Source: three-view drawing plus pictorial views. Frame: mm from the lowest corner of the part. Coordinates: 2 decimals unless noted, no trailing zeros. Loops run counter-clockwise (first coordinate to the right, second up) from the corner with the lowest first, then second, coordinate; pieces in that order, holes last. Notation, with made-up numbers: (59.5, 7) - (67.5, 7) arc R12 ccw to (67.5, 30) - close; hole circle Ø8 at (33.5, 15). An arc over 180 degrees is marked (long way). Return JSON: item names as keys, results as strings.
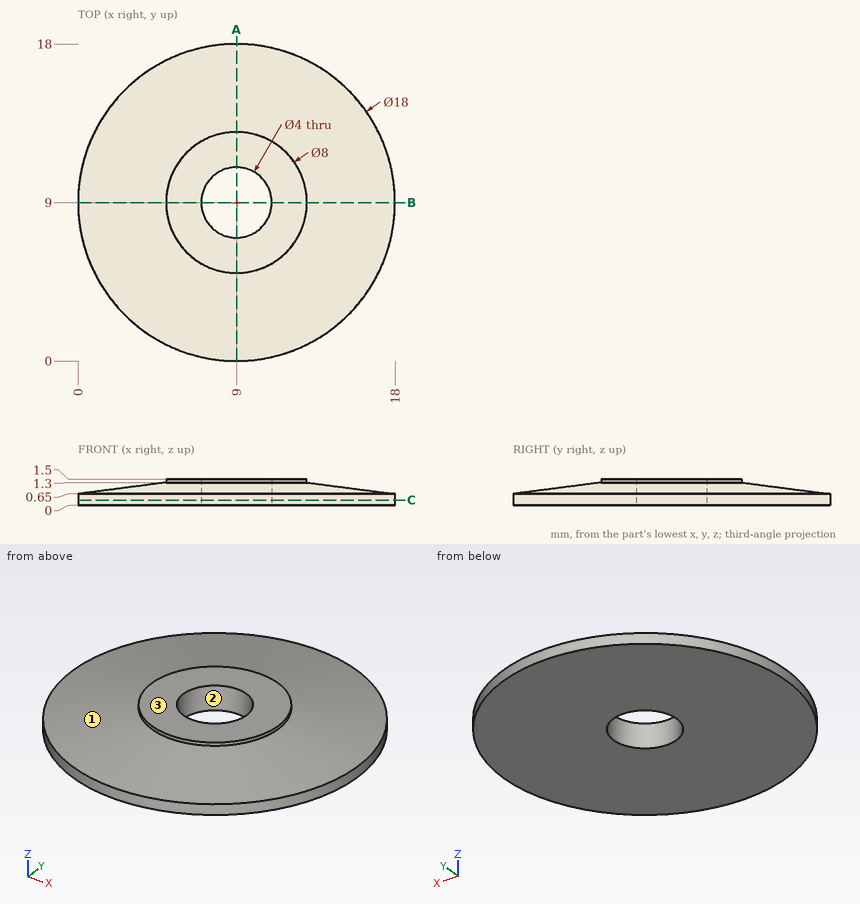
Item 1: Section query A-A, the plane x = 9. Return loops of the section in (y, z), and give its area (4 significant figures).
Worked out:
{"outline": "(0, 0) - (7, 0) - (7, 1.5) - (5, 1.5) - (5, 1.3) - (0, 0.65) - close; (11, 0) - (18, 0) - (18, 0.65) - (13, 1.3) - (13, 1.5) - (11, 1.5) - close", "area": "15.75 mm^2"}
Item 2: Ray query, probe 1 along Y at (x, z) = (10.5, 0.2); probe 2 along Z at (x, y) = (1.25, 13.5); probe 3 along Z at (x, y) = (1.25, 8.5). Return the intervals inside material, ascending. Write a range as from..to.
Worked out:
{"probe 1": "0.13..7.68, 10.32..17.87", "probe 2": "0..0.65", "probe 3": "0..0.81"}
Item 3: Mould query, pull axis Y, two halves, no side actions, for the marked faces 1, 2 and 3. Classes: +Y half, -Y half, draft (parallel to the pull), parting line (faces both ways), or undercut.
Worked out:
{"face 1": "parting line", "face 2": "undercut", "face 3": "draft"}
Item 4: Section query C-C, the plane z = 0.3. Return loops of the section in (x, y), and give its area (3 significant figures).
Worked out:
{"outline": "circle Ø18 at (9, 9); hole circle Ø4 at (9, 9)", "area": "242 mm^2"}
Item 5: First-contact query: pin 1 Ø8 at (x, y) = (11, 2) entering from +Z; pin 2 Ø1 at (x, y) = (14.5, 4.5) entering from +Z. Flat tips, straight axial feed; report the tip coordinate or a pass-through.
Worked out:
{"pin 1": "z = 1.5", "pin 2": "z = 0.96"}
